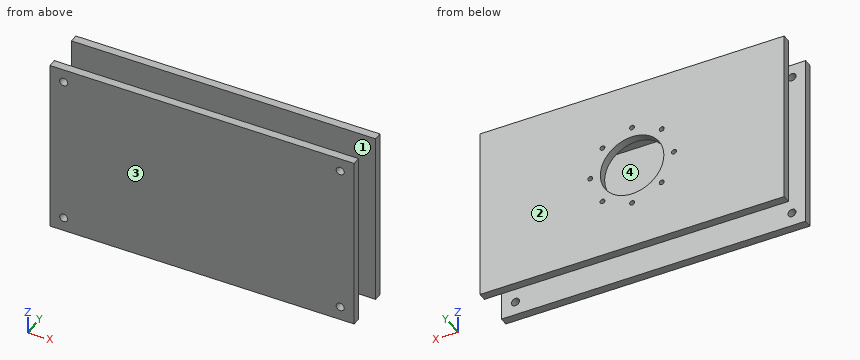
from build123d import *

# Parameters (mm, degrees)
SKETCH1_W           = 112.522
SKETCH1_H           = 66.04
SKETCH1_R           = 1.5
BOSS_EXTRUDE1_DEPTH = 3
SKETCH4_W           = 91.948
SKETCH4_H           = 44.704
BOSS_EXTRUDE2_DEPTH = 12
SHELL1_T            = -2.54
SKETCH13_R          = 3.253406585
CUT_EXTRUDE1_DEPTH  = 8.19
SKETCH15_R          = 3.393829234
CUT_EXTRUDE2_DEPTH  = 8.19
SKETCH16_W          = 112.522
SKETCH16_H          = 66.04
SKETCH16_R          = 11.75
SKETCH16_R_2        = 0.902882747
BOSS_EXTRUDE4_DEPTH = 3


with BuildPart() as part:
    # Sketch1 → Boss-Extrude1 (new body)
    with BuildSketch(Plane(origin=(0, 0, 0), x_dir=(1, 0, 0), z_dir=(0, 1, 0))):
        with Locations((4.991983213, -7.115654676)):
            Rectangle(SKETCH1_W, SKETCH1_H)
        with Locations(Location((-46.207741765, 20.726518927, 0), (0, 0, 270))):
            Circle(SKETCH1_R, mode=Mode.SUBTRACT)
        with Locations(Location((56.100367261, 20.726518927, 0), (0, 0, 270))):
            Circle(SKETCH1_R, mode=Mode.SUBTRACT)
        with Locations(Location((56.100367261, -35.155923699, 0), (0, 0, 270))):
            Circle(SKETCH1_R, mode=Mode.SUBTRACT)
        with Locations(Location((-46.207741765, -35.155923699, 0), (0, 0, 270))):
            Circle(SKETCH1_R, mode=Mode.SUBTRACT)
    extrude(amount=BOSS_EXTRUDE1_DEPTH)

    # Sketch4 → Boss-Extrude2 (add)
    with BuildSketch(Plane(origin=(0, 3, 0), x_dir=(1, 0, 0), z_dir=(0, 1, 0))):
        with Locations((4.991983213, -7.115654676)):
            Rectangle(SKETCH4_W, SKETCH4_H)
    extrude(amount=BOSS_EXTRUDE2_DEPTH)

    # Shell1
    shell1_openings = [part.faces().sort_by_distance(p)[0] for p in [
        (4.991983213, 15, 7.115654676),
    ]]
    offset(amount=SHELL1_T, openings=shell1_openings, kind=Kind.INTERSECTION)

    # Sketch13 → Cut-Extrude1 (cut)
    with BuildSketch(Plane.XY.offset(29.467654676)):
        with Locations((-28.892784248, 9.118527178)):
            Circle(SKETCH13_R)
    extrude(amount=-CUT_EXTRUDE1_DEPTH, mode=Mode.SUBTRACT)

    # Sketch15 → Cut-Extrude2 (cut)
    with BuildSketch(Plane.ZY.offset(40.982016787)):
        with Locations((-6.693412029, 8.197427611)):
            Circle(SKETCH15_R)
    extrude(amount=-CUT_EXTRUDE2_DEPTH, mode=Mode.SUBTRACT)

    # Sketch16 → Boss-Extrude4 (add)
    with BuildSketch(Plane(origin=(0, 15, 0), x_dir=(1, 0, 0), z_dir=(0, 1, 0))):
        with Locations((4.991983213, -7.115654676)):
            Rectangle(SKETCH16_W, SKETCH16_H)
        with Locations(Location((4.991983213, -7.115654676, 0), (0, 0, 270))):
            Circle(SKETCH16_R, mode=Mode.SUBTRACT)
        with Locations(Location((4.991983213, 8.384345324, 0), (0, 0, 270))):
            Circle(SKETCH16_R_2, mode=Mode.SUBTRACT)
        with Locations(Location((-5.968171895, 3.844500432, 0), (0, 0, 270))):
            Circle(SKETCH16_R_2, mode=Mode.SUBTRACT)
        with Locations(Location((-10.508016787, -7.115654676, 0), (0, 0, 270))):
            Circle(SKETCH16_R_2, mode=Mode.SUBTRACT)
        with Locations(Location((-5.968171895, -18.075809785, 0), (0, 0, 270))):
            Circle(SKETCH16_R_2, mode=Mode.SUBTRACT)
        with Locations(Location((4.991983213, -22.615654676, 0), (0, 0, 270))):
            Circle(SKETCH16_R_2, mode=Mode.SUBTRACT)
        with Locations(Location((15.952138322, -18.075809785, 0), (0, 0, 270))):
            Circle(SKETCH16_R_2, mode=Mode.SUBTRACT)
        with Locations(Location((20.491983213, -7.115654676, 0), (0, 0, 270))):
            Circle(SKETCH16_R_2, mode=Mode.SUBTRACT)
        with Locations(Location((15.952138322, 3.844500432, 0), (0, 0, 270))):
            Circle(SKETCH16_R_2, mode=Mode.SUBTRACT)
    extrude(amount=BOSS_EXTRUDE4_DEPTH)


solid = part.part
Model file for the job. Use its own axes, mm. Face numbers are marked on the shaded views. A direction names the side the tool comes from. Give positions to 0.01 mm unless a question says otherwise; leave off trailing zeros. Order: outer loops, then holes, each group sorted by start corner. A loop starts at its lowest first (then second) coordinate and runs counter-clockwise, first axis right, second up. Notation, with made-up numbers: (5, -14) - (34, -14) arc R25 ccw to (34, 2) - close; hole circle Ø1 at (3, -12). An arc over 180 degrees is marked (long way). One line per item, written item: value.
Item 1: Pin check, flat tips, straight feed: pin 1 Ø1.6 at (x, z) = (15.95, 18.08) entering from +Y; pin 2 Ø3.5 at (x, y) = (3, 7) entering from +Z; pin 3 Ø6 at (y, z) = (11, 1.5) entering from -X. Stop position of each tip, or through.
Response values:
pin 1: y = 2.54
pin 2: z = 29.47
pin 3: x = -40.98
Item 2: Two-plate mould, pull along Z, no slides. Class the marked faces 3 and 4: released by +Z, released by -Z, zero draft, split by the parting line, or undercut.
Response values:
face 3: zero draft
face 4: undercut
Item 3: Slice it at B-B (z = 1). List the corners of the cut face in (x, y) (3 decimals), then the cut area to 3 significant figures.
Response values:
outline: (-51.269, 0) - (61.253, 0) - (61.253, 3) - (50.966, 3) - (50.966, 15) - (61.253, 15) - (61.253, 18) - (15.025, 18) - (15.025, 15) - (48.426, 15) - (48.426, 2.54) - (-38.442, 2.54) - (-38.442, 15) - (-5.041, 15) - (-5.041, 18) - (-51.269, 18) - (-51.269, 15) - (-40.982, 15) - (-40.982, 3) - (-51.269, 3) - close
area: 636 mm2
Item 4: Wall check: line 1 (Z direction, x = 39.5, y = 9.75); line 2 (Y direction, x = -8.5, z = 1); line 3 (Y direction, x = -45, z = 24). Give the ranges that are in metal, low to high.
Response values:
line 1: -15.24 to -12.7, 26.93 to 29.47
line 2: 0 to 2.54, 15 to 18
line 3: 0 to 3, 15 to 18
Item 5: Slice it at A-A (x = -43.5). List the corners of the cut face in (y, z).
Response values:
outline: (0, -25.9) - (3, -25.9) - (3, 40.14) - (0, 40.14) - close; (15, -25.9) - (18, -25.9) - (18, 40.14) - (15, 40.14) - close
Item 6: Tool access for the marked faces 1 and 2: list every direction of +Z, -Z, +X, -X, +Y, -Y with a clear straight run to the whole face (end or side of a thin tool).
Response values:
face 1: none
face 2: +Z, -Z, +X, -X, +Y
